from build123d import *

# Parameters (mm, degrees)
BOSS_EXTRUDE1_DEPTH = 24
SKETCH1_4_R         = 28
SKETCH1_4_R_2       = 16
BOSS_EXTRUDE2_DEPTH = 56
SKETCH2_W           = 38.610961688
SKETCH2_H           = 6
CUT_EXTRUDE1_DEPTH  = 57
SKETCH3_R           = 16
CUT_EXTRUDE2_DEPTH  = 40


with BuildPart() as part:
    # Sketch1 → Boss-Extrude1 (new body)
    with BuildSketch(Plane(origin=(0, 0, 0), x_dir=(1, 0, 0), z_dir=(0, 1, 0))):
        with BuildLine():
            ThreePointArc((28, 24), (24.37028665, 10.212718594), (14.422205102, 0))
            Line((14.422205102, 0), (90, 0))
            Line((90, 0), (90, 48))
            Line((90, 48), (14.422205102, 48))
            ThreePointArc((14.422205102, 48), (24.37028665, 37.787281406), (28, 24))
        make_face()
    extrude(amount=BOSS_EXTRUDE1_DEPTH)

    # Sketch1_4 → Boss-Extrude2 (add)
    with BuildSketch(Plane(origin=(0, 0, 0), x_dir=(1, 0, 0), z_dir=(0, 1, 0))):
        with Locations((0, 24)):
            Circle(SKETCH1_4_R)
        with Locations((0, 24)):
            Circle(SKETCH1_4_R_2, mode=Mode.SUBTRACT)
    extrude(amount=BOSS_EXTRUDE2_DEPTH)

    # Sketch2 → Cut-Extrude1 (cut, through all)
    with BuildSketch(Plane(origin=(0, 56, 0), x_dir=(1, 0, 0), z_dir=(0, 1, 0))):
        with Locations((-21.356464049, 24.552208475)):
            Rectangle(SKETCH2_W, SKETCH2_H)
    extrude(amount=-CUT_EXTRUDE1_DEPTH, mode=Mode.SUBTRACT)

    # Sketch3 → Cut-Extrude2 (cut)
    with BuildSketch(Plane(origin=(90, 0, 0), x_dir=(0, 0, -1), z_dir=(1, 0, 0))):
        with Locations((24, 24)):
            Circle(SKETCH3_R)
    extrude(amount=-CUT_EXTRUDE2_DEPTH, mode=Mode.SUBTRACT)


solid = part.part
Design review of the part built by this model. Coordinates are the model's own, in mm. A direction names the side the tool comes from. Give positions to 0.01 mm unless a question says otherwise; leave off trailing zeros. Loops run counter-clockwise (first coordinate to the right, second up) from the corner with the lowest first, then second, coordinate; pieces in that order, holes last. Notation, with made-up numbers: (48, 32.25) - (66, 32.25) arc R32 ccw to (66, 65.25) - close; hole circle Ø10 at (79.5, -27). An arc over 180 degrees is marked (long way). Write item = value, one per line.
1) Take a section at A-A on x = 0. State the section outline as (y, z) points, and give its area (3 significant figures).
Result sheet:
outline = (0, -52) - (56, -52) - (56, -40) - (0, -40) - close; (0, -8) - (56, -8) - (56, 4) - (0, 4) - close
area = 1,340 mm2
2) Clearance check with flat-ended pins moving along their axes: pin 1 Ø10 at (y, z) = (15, -45.5) entering from -X; pin 2 Ø19 at (x, y) = (36.5, 6.5) entering from +Z; pin 3 Ø1 at (y, z) = (42.5, -7) entering from +X. State where each tip first meets the part, or that it passes through.
Result sheet:
pin_1 = -22.62
pin_2 = 0
pin_3 = 22.62
3) Draft analysis for pull direction X (two halves, no side actions). For faces 6 (the face through (15.953, 27.608, -22.777)), 7 (the face through (70, 8, -24)), 8 (the face through (-24.48, 27.61, -37.59)), 9 (the face through (50, 18, -24)), state which applies: +X half, -X half, draft (parallel to the pull), parting line (faces both ways), or undercut.
Result sheet:
face_6 = undercut
face_7 = draft
face_8 = parting line
face_9 = +X half
4) Take a section at D-D on x = 33. State the section outline as (y, z) points.
Result sheet:
outline = (0, -48) - (24, -48) - (24, 0) - (0, 0) - close
5) To check wall thickness, follow line 1 (Z direction, x = -0.5, y = 15.5); line 2 (X direction, y = 15.5, z = -24); line 3 (X direction, y = 38, z = -24). State the ranges of each line that lie inside material, in increasing order.
Result sheet:
line_1 = -52 to -39.99, -8.01 to 4
line_2 = 16 to 50
line_3 = 16 to 28
6) Take a section at C-C on z = -24. State the section outline as (x, y) points.
Result sheet:
outline = (16, 0) - (90, 0) - (90, 8) - (50, 8) - (50, 24) - (28, 24) - (28, 56) - (16, 56) - close
7) Tool access review of faces 1 (the face through (53, 12, -48)), 2 (the face through (-22, 28, -27.552)), 3 (the face through (30, 0, -24)), 4 (the face through (52, 12, 0)), 5 (the face through (12, 56, -12)): name each direction out of +Z, -Z, +X, -X, +Y, -Y from which nothing blocks a thin tool from reaching the whole face with its end or side.
Result sheet:
face_1 = -Z, +X, +Y, -Y
face_2 = -X, +Y, -Y
face_3 = +Z, -Z, +X, -X, -Y
face_4 = +Z, +X, +Y, -Y
face_5 = +Z, -Z, +X, -X, +Y
8) Take a section at B-B on z = -31. State the section outline as (x, y) points.
Result sheet:
outline = (-27.11, 0) - (-14.39, 0) - (-14.39, 56) - (-27.11, 56) - close; (14.39, 0) - (90, 0) - (90, 9.61) - (50, 9.61) - (50, 24) - (27.11, 24) - (27.11, 56) - (14.39, 56) - close
